from build123d import *

# Parameters (mm, degrees)
F0_W     = 1.27
F0_H     = 19.05
F1_DEPTH = 1.27
F2_W     = 6.94944
F2_H     = 1.27
F3_DEPTH = 1.27
F4_W     = 6.94944
F4_H     = 5.842
F5_DEPTH = 0.762


with BuildPart() as f1:
    # F0 (on Top) → F1 (new body)
    with BuildSketch(Plane.XY):
        with Locations((-2.83972, -2.891212)):
            Rectangle(F0_W, F0_H)
        with Locations((2.83972, -2.891212)):
            Rectangle(F0_W, F0_H)
    extrude(amount=F1_DEPTH)

    # F2 (on face) → F3 (join)
    with BuildSketch(Plane.XY.offset(1.27)):
        with Locations((0, 5.998788)):
            Rectangle(F2_W, F2_H)
        with Locations((0, 4.474788)):
            Rectangle(F2_W, F2_H)
        with Locations((0, 2.950788)):
            Rectangle(F2_W, F2_H)
        with Locations((0, 1.426788)):
            Rectangle(F2_W, F2_H)
        with Locations((0, -2.51257)):
            Rectangle(F2_W, F2_H)
        with Locations((0, -6.451929)):
            Rectangle(F2_W, F2_H)
    extrude(amount=F3_DEPTH)

    # F4 (on face) → F5 (join)
    with BuildSketch(Plane.XY.offset(1.27)):
        with Locations((0, 3.712788)):
            Rectangle(F4_W, F4_H)
    extrude(amount=F5_DEPTH)


solid = f1.part
Geometry: final body of the model. Coordinates: model frame, mm. A direction names the side the tool comes from. Give positions to 0.01 mm unless a question says otherwise; leave off trailing zeros. Order: outer loops, then holes, each group sorted by start corner. A loop starts at its lowest first (then second) coordinate and runs counter-clockwise, first axis right, second up. Notation, with made-up numbers: (33.5, -2.75) -> (70.5, -2.75) arc R10 ccw to (70.5, 16.25) -> close; hole circle Ø3 at (10.5, -37.75). An arc over 180 degrees is marked (long way). Answer as a JSON object with one key per item and string values.
Q1. Access query for faces 1 (the flat face through (2.205, -3, 1)), 2 (the flat face through (0, -5.817, 2)), 3 (the flat face through (-3, -10, 1.27)), 4 (the flat face through (-3, -3, 0)). Directions: +Z, -Z, +X, -X, +Y, -Y. A direction counts if a zero-diameter tool reaches every point of the face in a straight line with its end or side. Return the directions, or none.
Entries:
{"face 1": "-Z, +Y, -Y", "face 2": "+Z, +X, -X", "face 3": "+Z, +X, -X, -Y", "face 4": "-Z, +X, -X, +Y, -Y"}
Q2. Section A-A (x = -1). Output: boundary loops of the cut face in (y, z).
Entries:
{"outline": "(-7.09, 1.27) -> (-5.82, 1.27) -> (-5.82, 2.54) -> (-7.09, 2.54) -> close; (-3.15, 1.27) -> (-1.88, 1.27) -> (-1.88, 2.54) -> (-3.15, 2.54) -> close; (0.79, 1.27) -> (6.63, 1.27) -> (6.63, 2.54) -> (5.36, 2.54) -> (5.36, 2.03) -> (5.11, 2.03) -> (5.11, 2.54) -> (3.84, 2.54) -> (3.84, 2.03) -> (3.59, 2.03) -> (3.59, 2.54) -> (2.32, 2.54) -> (2.32, 2.03) -> (2.06, 2.03) -> (2.06, 2.54) -> (0.79, 2.54) -> close"}
Q3. Section D-D (z = 0.3). Output: boundary loops of the cut face in (x, y), plus the area to 3 significant figures.
Entries:
{"outline": "(-3.47, -12.42) -> (-2.2, -12.42) -> (-2.2, 6.63) -> (-3.47, 6.63) -> close; (2.2, -12.42) -> (3.47, -12.42) -> (3.47, 6.63) -> (2.2, 6.63) -> close", "area": "48.4 mm^2"}
Q4. Section B-B (z = 1.6). Output: boundary loops of the cut face in (x, y).
Entries:
{"outline": "(-3.47, -7.09) -> (3.47, -7.09) -> (3.47, -5.82) -> (-3.47, -5.82) -> close; (-3.47, -3.15) -> (3.47, -3.15) -> (3.47, -1.88) -> (-3.47, -1.88) -> close; (-3.47, 0.79) -> (3.47, 0.79) -> (3.47, 6.63) -> (-3.47, 6.63) -> close"}
Q5. First-contact query: pin 1 (1.4 mm diameter, centred on x = -1, y = -2.5, fed in from -Z); pin 2 (1 mm diameter, centred on x = -1.5, z = 2, fed in from -Y); pin 3 (1.4 mm diameter, centred on x = -3, y = -4, fed in from +Z). Flat tips, straight axial feed; report the tip coordinate or a pass-through.
Entries:
{"pin 1": "stops at z = 1.27", "pin 2": "stops at y = -7.09", "pin 3": "stops at z = 1.27"}
Q6. Section C-C (y = -0.75). Output: boundary loops of the cut face in (x, z), plus the area to 3 significant figures.
Entries:
{"outline": "(-3.47, 0) -> (-2.2, 0) -> (-2.2, 1.27) -> (-3.47, 1.27) -> close; (2.2, 0) -> (3.47, 0) -> (3.47, 1.27) -> (2.2, 1.27) -> close", "area": "3.23 mm^2"}
Q7. Material intervals for probe 1 along Y at (x, z) = (0.25, 2.45); probe 2 along Y at (x, z) = (-2.25, 1.45); probe 3 along X at (y, z) = (-1, 0.8), sorted ascending.
Entries:
{"probe 1": "y = -7.09 to -5.82, -3.15 to -1.88, 0.79 to 2.06, 2.32 to 3.59, 3.84 to 5.11, 5.36 to 6.63", "probe 2": "y = -7.09 to -5.82, -3.15 to -1.88, 0.79 to 6.63", "probe 3": "x = -3.47 to -2.2, 2.2 to 3.47"}
Q8. Draft query along Y for faces 5 (the flat face through (0, -1.878, 2)), 6 (the flat face through (0, -2.5, 1.27)), 7 (the flat face through (-3, -12.416, 1)). Return one class per face: released by +Y, released by -Y, zero draft, split by the parting line, or undercut.
Entries:
{"face 5": "undercut", "face 6": "zero draft", "face 7": "released by -Y"}
